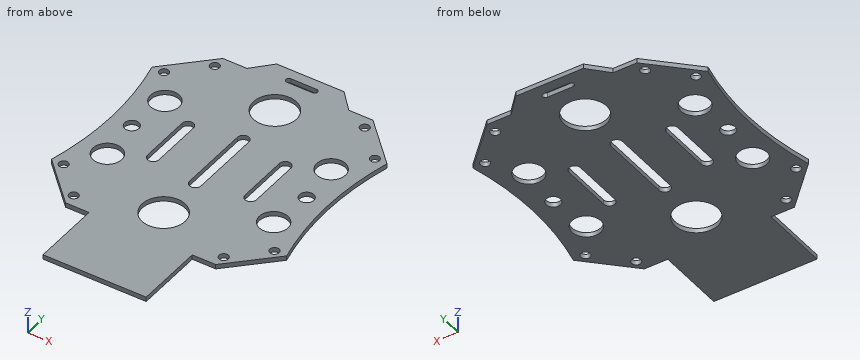
```python
from build123d import *

# Parameters (mm, degrees)
F0_R     = 1.625
F0_R_2   = 5
F0_R_3   = 7.5
F0_R_4   = 2.5
F1_DEPTH = 1.6002


with BuildPart() as f1:
    # F0 (on Top) → F1 (new body)
    with BuildSketch(Plane.XY):
        with BuildLine():
            Line((11.75, 47.5), (-11.75, 47.5))
            Line((-11.75, 47.5), (-17.75, 41))
            Line((-17.75, 41), (-26.175144, 41))
            Line((-26.175144, 41), (-41, 26.175144))
            ThreePointArc((-41, 26.175144), (-37.75, 0), (-41, -26.175144))
            Line((-41, -26.175144), (-26.175144, -41))
            Line((-26.175144, -41), (-18, -41))
            Line((-18, -41), (-18, -65))
            Line((-18, -65), (18, -65))
            Line((18, -65), (18, -41))
            Line((18, -41), (26.175144, -41))
            Line((26.175144, -41), (41, -26.175144))
            ThreePointArc((41, -26.175144), (37.75, 0), (41, 26.175144))
            Line((41, 26.175144), (26.175144, 41))
            Line((26.175144, 41), (17.75, 41))
            Line((17.75, 41), (11.75, 47.5))
        make_face()
        with Locations((-36.769553, -26.162951)):
            Circle(F0_R, mode=Mode.SUBTRACT)
        with Locations((-26.162951, -36.769553)):
            Circle(F0_R, mode=Mode.SUBTRACT)
        with Locations((-29, -15)):
            Circle(F0_R_2, mode=Mode.SUBTRACT)
        with Locations((0, -29)):
            Circle(F0_R_3, mode=Mode.SUBTRACT)
        with Locations((26.162951, -36.769553)):
            Circle(F0_R, mode=Mode.SUBTRACT)
        with Locations((36.769553, -26.162951)):
            Circle(F0_R, mode=Mode.SUBTRACT)
        with Locations((29, -15)):
            Circle(F0_R_2, mode=Mode.SUBTRACT)
        with Locations((-30.5, 0)):
            Circle(F0_R_4, mode=Mode.SUBTRACT)
        with Locations((-29, 15)):
            Circle(F0_R_2, mode=Mode.SUBTRACT)
        with BuildLine():
            Line((-19, -9), (-19, 9))
            ThreePointArc((-19, 9), (-17, 11), (-15, 9))
            Line((-15, 9), (-15, -9))
            ThreePointArc((-15, -9), (-17, -11), (-19, -9))
        make_face(mode=Mode.SUBTRACT)
        with Locations((-36.769553, 26.162951)):
            Circle(F0_R, mode=Mode.SUBTRACT)
        with Locations((-26.162951, 36.769553)):
            Circle(F0_R, mode=Mode.SUBTRACT)
        with BuildLine():
            Line((-2, -12.5), (-2, 12.5))
            ThreePointArc((-2, 12.5), (0, 14.5), (2, 12.5))
            Line((2, 12.5), (2, -12.5))
            ThreePointArc((2, -12.5), (0, -14.5), (-2, -12.5))
        make_face(mode=Mode.SUBTRACT)
        with BuildLine():
            Line((19, 9), (19, -9))
            ThreePointArc((19, -9), (17, -11), (15, -9))
            Line((15, -9), (15, 9))
            ThreePointArc((15, 9), (17, 11), (19, 9))
        make_face(mode=Mode.SUBTRACT)
        with Locations((30.5, 0)):
            Circle(F0_R_4, mode=Mode.SUBTRACT)
        with Locations((29, 15)):
            Circle(F0_R_2, mode=Mode.SUBTRACT)
        with Locations((0, 29)):
            Circle(F0_R_3, mode=Mode.SUBTRACT)
        with BuildLine():
            ThreePointArc((-4.5, 42), (-5.5, 43), (-4.5, 44))
            Line((-4.5, 44), (4.5, 44))
            ThreePointArc((4.5, 44), (5.5, 43), (4.5, 42))
            Line((4.5, 42), (-4.5, 42))
        make_face(mode=Mode.SUBTRACT)
        with Locations((36.769553, 26.162951)):
            Circle(F0_R, mode=Mode.SUBTRACT)
        with Locations((26.162951, 36.769553)):
            Circle(F0_R, mode=Mode.SUBTRACT)
    extrude(amount=F1_DEPTH)


solid = f1.part
```
Can you work these out from the model? Positions are in its coordinate system, mm. Round coordinates to 2 decimals unless told otherwise and drop trailing zeros. Loops run counter-clockwise (first coordinate to the right, second up) from the corner with the lowest first, then second, coordinate; pieces in that order, holes last. Notation, with made-up numbers: (-16, 12) -> (15, 12) arc R14 ccw to (15, 20) -> close; hole circle Ø3 at (52.5, 35.25). An arc over 180 degrees is marked (long way). One line per item, written item: value. Start each with the question number.
1. If we section it at A-A, the plane y = -29: Write out the boundary of the cut face in (x, z), then the cut area to 3 significant figures.
2. For pin 1 (0.8 mm diameter, centred on y = -47.5, z = 1, fed in from -X); pin 2 (3 mm diameter, centred on x = 36.77, y = 26.16, fed in from -Z), each with a flat end and sliding along its axis, tell me the tip position at first contact or that it passes through.
3. If we section it at B-B, the plane z = 0.9: Give the number of separate pieces and of enclosed holes in the cut face, then the cut area to 3 significant figures.
4. If I drill on probe 1 along Y at (x, z) = (0, 1.15); probe 2 along X at (y, z) = (19, 1.3); probe 3 along X at (y, z) = (-2, 1.1), over which ranges is the centre line in solid material (lowest first)?
Calculated:
1. outline: (-38.18, 0) -> (-7.5, 0) -> (-7.5, 1.6) -> (-38.18, 1.6) -> close; (7.5, 0) -> (38.18, 0) -> (38.18, 1.6) -> (7.5, 1.6) -> close
1. area: 98.2 mm²
2. pin 1: stops at x = -18
2. pin 2: passes through
3. separate pieces: 1
3. enclosed holes: 20
3. area: 6,040 mm²
4. probe 1: y = -65 to -36.5, -21.5 to -14.5, 14.5 to 21.5, 36.5 to 42, 44 to 47.5
4. probe 2: x = -39.45 to -32, -26 to 26, 32 to 39.45
4. probe 3: x = -37.77 to -32, -29 to -19, -15 to -2, 2 to 15, 19 to 29, 32 to 37.77
